Could you check a few things on this model? Use its own coordinates, in mm. A direction names the side the tool comes from. Round coordinates to 2 decimals unless told otherwise and drop trailing zeros. Loops run counter-clockwise (first coordinate to the right, second up) from the corner with the lowest first, then second, coordinate; pieces in that order, holes last. Notation, with made-up numbers: M -28.75,27 L 7.25,27 A8 ccw 7.25,37 Z; hole C 86.25,-13.75 d4. An arc over 180 degrees is marked long. Return JSON: item names as keys, results as strings. Group by question number.
```python
from build123d import *

# Parameters (mm, degrees)
F0_W      = 2320
F0_H      = 630
F0_W_2    = 40
F0_H_2    = 446
F1_DEPTH  = 40
F2_W      = 40
F2_H      = 40
F3_DEPTH  = 40
F4_W      = 50
F4_H      = 5
F4_W_2    = 40
F5_DEPTH  = 40
F9_W      = 60
F9_H      = 40
F10_DEPTH = 5


# Not quite as in the source:
# - a feature names something its author has since deleted; it is built from what else it names


with BuildPart() as f1:
    # F0 (on Front) → F1 (new body)
    with BuildSketch(Plane.XZ):
        Polygon((1200, 432.3376794357), (-1200, 432.3376794357), (-1200, -277.6623205643), (-1160, -277.6623205643), (1160, -277.6623205643), (1200, -277.6623205643), align=None)
        with Locations((0, 77.3376794357)):
            Rectangle(F0_W, F0_H, mode=Mode.SUBTRACT)
        with Locations((1180, -500.6623205643)):
            Rectangle(F0_W_2, F0_H_2)
        with Locations((-1180, -500.6623205643)):
            Rectangle(F0_W_2, F0_H_2)
    extrude(amount=F1_DEPTH)

    # F2 (on face) → F3 (join)
    with BuildSketch(Plane(origin=(-1200, 0, 0), x_dir=(0, -1, 0), z_dir=(-1, 0, 0))):
        Polygon((40, -625.9272936454), (140, -683.6623205643), (220, -683.6623205643), (40, -579.7392721102), align=None)
        Polygon((0, -579.7392721102), (-180, -683.6623205643), (-100, -683.6623205643), (0, -625.9272936454), align=None)
        Polygon((-280, -683.6623205643), (-280, -723.6623205643), (0, -723.6623205643), (0, -683.6623205643), (-100, -683.6623205643), (-180, -683.6623205643), align=None)
        Polygon((40, -683.6623205643), (40, -723.6623205643), (320, -723.6623205643), (320, -683.6623205643), (220, -683.6623205643), (140, -683.6623205643), align=None)
        with Locations((20, -703.6623205643)):
            Rectangle(F2_W, F2_H)
    extrude(amount=-F3_DEPTH)

    # F4 (on face) → F5 (join)
    with BuildSketch(Plane.YZ.offset(-1160)):
        with Locations((25, -495.1623205643)):
            Rectangle(F4_W, F4_H)
        with Locations((-20, -495.1623205643)):
            Rectangle(F4_W_2, F4_H)
        with Locations((-65, -495.1623205643)):
            Rectangle(F4_W, F4_H)
    extrude(amount=F5_DEPTH)

    # F6: F1 across plane


with BuildPart() as f1_1:
    add(f1.part)
    add(f1.part.mirror(Plane.YZ))

    # F7: F1 across plane


with BuildPart() as f1_2:
    add(f1_1.part)
    add(f1_1.part.mirror(Plane.YZ))

    # F9 (on offset) → F10 (join)
    with BuildSketch(Plane.XZ.offset(20)):
        with Locations((-1130, -217.6623205643)):
            Rectangle(F9_W, F9_H)
        with Locations((-1130, 372.3376794357)):
            Rectangle(F9_W, F9_H)
        with Locations((-375, 372.3376794357)):
            Rectangle(F9_W, F9_H)
        with Locations((-375, -217.6623205643)):
            Rectangle(F9_W, F9_H)
        with Locations((375, -217.6623205643)):
            Rectangle(F9_W, F9_H)
        with Locations((375, 372.3376794357)):
            Rectangle(F9_W, F9_H)
        with Locations((1130, 372.3376794357)):
            Rectangle(F9_W, F9_H)
        with Locations((1130, -217.6623205643)):
            Rectangle(F9_W, F9_H)
    extrude(amount=F10_DEPTH)


solid = f1_2.part
```
1. I'm going to push flat-ended pins straight in: pin 1 Ø5.5 at (y, z) = (32, -495.5) entering from -X; pin 2 Ø12 at (x, y) = (1179, 30.5) entering from +Z; pin 3 Ø20 at (x, y) = (1174.5, 231.5) entering from +Z. Where does each tip first touch, or does it pass through?
2. I need wall thicknesses on probe 1 along X at (y, z) = (-9, 224); probe 2 along Z at (x, y) = (81, -18). Which ranges of each line are inside material? Lowest first, please.
3. On a 3-axis mill with a long thin cutter (end or side, diameter ignored), from which of +Z, -Z, +X, -X, +Y, -Y can I reach the whole of each face in a straight line? I mean faces 4 (the face through (1160, -16, -662)), 5 (the face through (-1180.28, 88.74, -630.973)). Say none if no direction works.
4. If we section it at A-A, the plane x = 853.5: Please give me the cut outline in (y, z), then the cut area to 3 significant figures.
5. If we section it at B-B, the plane z = -131: Please give me the cut outline in (x, y), then the cut area to 3 significant figures.
6. We'd pull the mould along Z, two halves only. Please class faces 1 (the face through (-1160, -16, -659)), 2 (the face through (-1180.28, -89.3, -654.39)), 3 (the face through (1180.28, 88.74, -630.973)): +Z half, -Z half, draft (parallel to the pull), parting line (faces both ways), or undercut.
Geometry results:
{
 "1": {"pin 1": "x = -1160", "pin 2": "z = -593.88", "pin 3": "z = -683.66"},
 "2": {"probe 1": "-1200 to -1160, 1160 to 1200", "probe 2": "-277.66 to -237.66, 392.34 to 432.34"},
 "3": {"face 4": "-Z, +Y, -Y", "face 5": "+Z, +X, -X, +Y"},
 "4": {"outline": "M -40,-277.66 L 0,-277.66 L 0,-237.66 L -40,-237.66 Z; M -40,392.34 L 0,392.34 L 0,432.34 L -40,432.34 Z", "area": "3,200 mm^2"},
 "5": {"outline": "M -1200,-40 L -1160,-40 L -1160,0 L -1200,0 Z; M 1160,-40 L 1200,-40 L 1200,0 L 1160,0 Z", "area": "3,200 mm^2"},
 "6": {"face 1": "draft", "face 2": "undercut", "face 3": "+Z half"}
}
